```python
from build123d import *

# Parameters (mm, degrees)
SKETCH1_W           = 19.9
SKETCH1_H           = 9.55
SKETCH1_R           = 1
BOSS_EXTRUDE1_DEPTH = 6.4
SKETCH2_R           = 1.575054
BOSS_EXTRUDE2_DEPTH = 0.8636
SKETCH3_R           = 1.575054
SKETCH3_R_2         = 0.79375
CUT_EXTRUDE1_DEPTH  = 0.381
SKETCH4_W           = 2.8
SKETCH4_H           = 0.5
BOSS_EXTRUDE3_DEPTH = 6.35
CHAMFER1_SIZE       = 0.889


with BuildPart() as part:
    # Sketch1 → Boss-Extrude1 (new body)
    with BuildSketch(Plane(origin=(0, 0, 0), x_dir=(1, 0, 0), z_dir=(0, 1, 0))):
        with Locations((9.95, 4.775)):
            Rectangle(SKETCH1_W, SKETCH1_H)
        with Locations((5.13, 2.35)):
            Circle(SKETCH1_R, mode=Mode.SUBTRACT)
        with Locations((14.66, 2.35)):
            Circle(SKETCH1_R, mode=Mode.SUBTRACT)
    extrude(amount=BOSS_EXTRUDE1_DEPTH)

    # Sketch2 → Boss-Extrude2 (add)
    with BuildSketch(Plane(origin=(0, 0, -9.55), x_dir=(-1, 0, 0), z_dir=(0, 0, -1))):
        with Locations((-7.1, 3.2)):
            Circle(SKETCH2_R)
    extrude(amount=BOSS_EXTRUDE2_DEPTH)

    # Sketch3 → Cut-Extrude1 (cut)
    with BuildSketch(Plane(origin=(0, 0, -10.4136), x_dir=(-1, 0, 0), z_dir=(0, 0, -1))):
        with Locations((-7.1, 3.2)):
            Circle(SKETCH3_R)
        with Locations((-7.1, 3.2)):
            Circle(SKETCH3_R_2, mode=Mode.SUBTRACT)
    extrude(amount=-CUT_EXTRUDE1_DEPTH, mode=Mode.SUBTRACT)

    # Sketch4 → Boss-Extrude3 (add)
    with BuildSketch(Plane.XY):
        with Locations((2.67, 3.2)):
            Rectangle(SKETCH4_W, SKETCH4_H)
        with Locations((9.95, 3.2)):
            Rectangle(SKETCH4_W, SKETCH4_H)
        with Locations((17.23, 3.2)):
            Rectangle(SKETCH4_W, SKETCH4_H)
    extrude(amount=BOSS_EXTRUDE3_DEPTH)

    # Chamfer1
    chamfer1_edges = [part.edges().sort_by_distance(p)[0] for p in [
        (1.27, 3.2, 6.35),
        (4.07, 3.2, 6.35),
        (8.55, 3.2, 6.35),
        (11.35, 3.2, 6.35),
        (15.83, 3.2, 6.35),
        (18.63, 3.2, 6.35),
    ]]
    chamfer(chamfer1_edges, length=CHAMFER1_SIZE)


solid = part.part
```
Source: CAD feature listing. Evaluate the final solid. Frame: model axes, mm. A direction names the side the tool comes from. Coordinates: 2 decimals unless noted, no trailing zeros. Loops run counter-clockwise (first coordinate to the right, second up) from the corner with the lowest first, then second, coordinate; pieces in that order, holes last. Notation, with made-up numbers: (-20, 88) -> (6, 88) arc R12 ccw to (6, 99) -> close; hole circle Ø8 at (40, 70). An arc over 180 degrees is marked (long way). One line per item, written item: value. Start each with the question number.
Q1. Line query: line 1 along X through (y, z) = (4, -2.35); line 2 along Z through (x, y) = (5.13, 4); line 3 along X through (y, z) = (3.5, -1.5). Output: solid intervals per line, ascending.
Q2. Section query B-B, the plane y = 3.2. Give the number of separate pieces and of enclosed holes in the cut face, and give its area (3 significant figures).
Q3. Section query C-C, the plane x = 14.66. Return the cut outline in (y, z).
Q4. Section query A-A, the plane z = 1.75. Return the cut outline in (x, y), and give its area (3 significant figures).
Q5. Section query D-D, the plane z = -2.35. Return the cut outline in (x, y).
Q6. Mould query, pull axis Z, two halves, no side actions, for faces 5 (the face through (13.66, 3.16, -2.39)), 6 (the face through (7, 3, -10.414)), 7 (the face through (3.62, 3.2, 5.91)). Classes: pulls with the +Z half, pulls with the -Z half, needs draft (parallel to the pull), parting line crosses it, or undercut.
Q7. Set-up query: faces 1 (the face through (3, 2.95, 3)), 2 (the face through (10.9, 3.2, 5.91)), 3 (the face through (10, 3.45, 3)), 4 (the face through (8, 4, -10.033)). Return all of +Z, -Z, +X, -X, +Y, -Y with unobstructed straight access to the full face (end or side cutting, diameter ignored); none if empty.
Q8. Contact query for flat-ended pins moving along their axis: P1, Ø0.6, axis at y = 3, z = 2.5, coming from the +X side; P2, Ø2, axis at x = 11, y = 5.5, coming from the +Z side; P3, Ø1.4, axis at x = 17.5, z = 3, coming from the -Y side. Output: stop coordinate, or through.
Results:
1. line 1: 0 to 4.13, 6.13 to 13.66, 15.66 to 19.9
1. line 2: -9.55 to -3.35, -1.35 to 0
1. line 3: 0 to 4.6, 5.66 to 14.13, 15.19 to 19.9
2. separate pieces: 1
2. enclosed holes: 2
2. area: 237 mm^2
3. outline: (0, -9.55) -> (6.4, -9.55) -> (6.4, -3.35) -> (0, -3.35) -> close; (0, -1.35) -> (6.4, -1.35) -> (6.4, 0) -> (0, 0) -> close
4. outline: (1.27, 2.95) -> (4.07, 2.95) -> (4.07, 3.45) -> (1.27, 3.45) -> close; (8.55, 2.95) -> (11.35, 2.95) -> (11.35, 3.45) -> (8.55, 3.45) -> close; (15.83, 2.95) -> (18.63, 2.95) -> (18.63, 3.45) -> (15.83, 3.45) -> close
4. area: 4.20 mm^2
5. outline: (0, 0) -> (4.13, 0) -> (4.13, 6.4) -> (0, 6.4) -> close; (6.13, 0) -> (13.66, 0) -> (13.66, 6.4) -> (6.13, 6.4) -> close; (15.66, 0) -> (19.9, 0) -> (19.9, 6.4) -> (15.66, 6.4) -> close
6. face 5: undercut
6. face 6: pulls with the -Z half
6. face 7: pulls with the +Z half
7. face 1: +Z, +X, -X, -Y
7. face 2: +Z, +Y, -Y
7. face 3: +Z, +X, -X, +Y
7. face 4: -Z
8. P1: x = 18.63
8. P2: z = 0
8. P3: y = 2.95
